```python
from build123d import *

# Parameters (mm, degrees)
SKETCH1_W                        = 125
SKETCH1_H                        = 120
TEST_BASE_POSTION_DEPTH          = 11.215
SKETCH8_R                        = 20.5
FINGER_GEARS_DEPTH               = 7
SKETCH9_R                        = 10.5
INTERMEDIATE_GEAR_DEPTH          = 7
SKETCH11_R                       = 18.5
XL320_FINGER_KNUCKLE_MOUNT_DEPTH = 7
SKETCH10_R                       = 15.5
CONNECT_FINGER_HOLES_DEPTH       = 88.361468766
THUMB_MOUNT_HOLES_R              = 2.25
THUMB_MOUNT_HOLES_M4_DEPTH       = 88.361468766
SKETCH16_R                       = 2.25
FINGERS_MOUNT_HOLES_M4_DEPTH     = 88.361468766
SKETCH17_R                       = 3.25
CONNECT_HOLES_M6_DEPTH           = 88.361468766
SKETCH18_R                       = 3.75
NUTS_M4_DEPTH                    = 4
SKETCH19_R                       = 5.25
NUTS_M6_DEPTH                    = 6


with BuildPart() as part:
    # Sketch1 → Test_Base_Postion (new body)
    with BuildSketch(Plane(origin=(0, 0, 0), x_dir=(1, 0, 0), z_dir=(0, 1, 0))):
        Rectangle(SKETCH1_W, SKETCH1_H)
    extrude(amount=TEST_BASE_POSTION_DEPTH)

    # Sketch8 → Finger_Gears (cut)
    with BuildSketch(Plane(origin=(0, 11.215, 0), x_dir=(1, 0, 0), z_dir=(0, 1, 0))):
        with Locations((-25.25, -19)):
            Circle(SKETCH8_R)
        with Locations((-25.25, 19)):
            Circle(SKETCH8_R)
    extrude(amount=-FINGER_GEARS_DEPTH, mode=Mode.SUBTRACT)

    # Sketch9 → Intermediate_Gear (cut)
    with BuildSketch(Plane(origin=(0, 11.215, 0), x_dir=(1, 0, 0), z_dir=(0, 1, 0))):
        with Locations((0.646123438, -8.351488795)):
            Circle(SKETCH9_R)
    extrude(amount=-INTERMEDIATE_GEAR_DEPTH, mode=Mode.SUBTRACT)

    # Sketch11 → XL320_Finger_Knuckle_Mount (cut)
    with BuildSketch(Plane(origin=(0, 11.215, 0), x_dir=(1, 0, 0), z_dir=(0, 1, 0))):
        with Locations(Location((42, 0, 0), (0, 0, 270))):
            Circle(SKETCH11_R)
    extrude(amount=-XL320_FINGER_KNUCKLE_MOUNT_DEPTH, mode=Mode.SUBTRACT)

    # Sketch10 → Connect_Finger_Holes (cut, through all)
    with BuildSketch(Plane(origin=(0, 11.215, 0), x_dir=(1, 0, 0), z_dir=(0, 1, 0))):
        with Locations(Location((-25.25, 19, 0), (0, 0, 270))):
            Circle(SKETCH10_R)
        with Locations(Location((-25.25, -19, 0), (0, 0, 270))):
            Circle(SKETCH10_R)
        with Locations(Location((42, 0, 0), (0, 0, 270))):
            Circle(SKETCH10_R)
    extrude(amount=-CONNECT_FINGER_HOLES_DEPTH, mode=Mode.SUBTRACT)

    # Thumb_Mount_Holes → Thumb_Mount_Holes_(M4) (cut, through all)
    with BuildSketch(Plane(origin=(0, 11.215, 0), x_dir=(1, 0, 0), z_dir=(0, 1, 0))):
        with Locations(Location((21.5, 44.5, 0), (0, 0, 270))):
            Circle(THUMB_MOUNT_HOLES_R)
        with Locations(Location((42, 53.5, 0), (0, 0, 270))):
            Circle(THUMB_MOUNT_HOLES_R)
        with Locations(Location((48, -24, 0), (0, 0, 270))):
            Circle(THUMB_MOUNT_HOLES_R)
        with Locations(Location((36, -24, 0), (0, 0, 270))):
            Circle(THUMB_MOUNT_HOLES_R)
    extrude(amount=-THUMB_MOUNT_HOLES_M4_DEPTH, mode=Mode.SUBTRACT)

    # Sketch16 → Fingers_Mount_Holes_(M4) (cut, through all)
    with BuildSketch(Plane(origin=(0, 11.215, 0), x_dir=(1, 0, 0), z_dir=(0, 1, 0))):
        with Locations(Location((11.5, 41, 0), (0, 0, 270))):
            Circle(SKETCH16_R)
        with Locations(Location((11.5, -41, 0), (0, 0, 270))):
            Circle(SKETCH16_R)
        with Locations(Location((-53, 6, 0), (0, 0, 270))):
            Circle(SKETCH16_R)
        with Locations(Location((-53, -6, 0), (0, 0, 270))):
            Circle(SKETCH16_R)
    extrude(amount=-FINGERS_MOUNT_HOLES_M4_DEPTH, mode=Mode.SUBTRACT)

    # Sketch17 → Connect_Holes_(M6) (cut, through all)
    with BuildSketch(Plane(origin=(0, 11.215, 0), x_dir=(1, 0, 0), z_dir=(0, 1, 0))):
        with Locations(Location((-52.5, 50, 0), (0, 0, 270))):
            Circle(SKETCH17_R)
        with Locations(Location((-52.5, -50, 0), (0, 0, 270))):
            Circle(SKETCH17_R)
        with Locations(Location((52.5, -50, 0), (0, 0, 270))):
            Circle(SKETCH17_R)
    extrude(amount=-CONNECT_HOLES_M6_DEPTH, mode=Mode.SUBTRACT)

    # Sketch18 → Nuts_(M4) (cut)
    with BuildSketch(Plane.XZ):
        with Locations(Location((11.5, 41, 0), (0, 0, 270))):
            Circle(SKETCH18_R)
        with Locations(Location((11.5, -41, 0), (0, 0, 270))):
            Circle(SKETCH18_R)
        with Locations(Location((21.5, -44.5, 0), (0, 0, 270))):
            Circle(SKETCH18_R)
        with Locations(Location((42, -53.5, 0), (0, 0, 270))):
            Circle(SKETCH18_R)
    extrude(amount=-NUTS_M4_DEPTH, mode=Mode.SUBTRACT)

    # Sketch19 → Nuts_(M6) (cut)
    with BuildSketch(Plane.XZ):
        with Locations(Location((-52.5, 50, 0), (0, 0, 270))):
            Circle(SKETCH19_R)
        with Locations(Location((52.5, 50, 0), (0, 0, 270))):
            Circle(SKETCH19_R)
        with Locations(Location((-52.5, -50, 0), (0, 0, 270))):
            Circle(SKETCH19_R)
    extrude(amount=-NUTS_M6_DEPTH, mode=Mode.SUBTRACT)


solid = part.part
```
Check sheet for the modelled part. Datum: model origin and axes. Units: mm. A direction names the side the tool comes from. Round coordinates to 2 decimals unless told otherwise and drop trailing zeros. Loops run counter-clockwise (first coordinate to the right, second up) from the corner with the lowest first, then second, coordinate; pieces in that order, holes last. Notation, with made-up numbers: M 52,21.5 L 86,21.5 A21 cw 86,27.5 Z; hole C 2.25,52.5 d3. An arc over 180 degrees is marked long. Answer as a JSON object with one key per item and string values.
1. Section check D-D (y = 7.5). State how many separate pieces and enclosed holes the cut face has, plus the area to 3 significant figures.
Reply:
{"separate pieces": "1", "enclosed holes": "13", "area": "10,800 mm²"}
2. Section check C-C (x = -25.25). Record the boundary of the cut face in (y, z) (3 decimals).
Reply:
{"outline": "M 0,-60 L 11.215,-60 L 11.215,-39.5 L 4.215,-39.5 L 4.215,-34.5 L 0,-34.5 Z; M 0,-3.5 L 4.215,-3.5 L 4.215,3.5 L 0,3.5 Z; M 0,34.5 L 4.215,34.5 L 4.215,39.5 L 11.215,39.5 L 11.215,60 L 0,60 Z"}
3. Scan lines: line 1 (X direction, y = 7.85, z = 50); line 2 (Z direction, x = -26, y = 2.75); line 3 (X direction, y = 3.2, z = -19). Record each from-to range of solid material in increasing order.
Reply:
{"line 1": "x = -62.5 to -55.75, -49.25 to 49.25, 55.75 to 62.5", "line 2": "z = -60 to -34.48, -3.52 to 3.52, 34.48 to 60", "line 3": "x = -62.5 to -40.75, -9.75 to 62.5"}
4. Section check B-B (z = 41). Record the boundary of the cut face in (x, y) (3 decimals).
Reply:
{"outline": "M -62.5,0 L 7.75,0 L 7.75,4 L 9.25,4 L 9.25,11.215 L -62.5,11.215 Z; M 13.75,4 L 15.25,4 L 15.25,0 L 62.5,0 L 62.5,11.215 L 13.75,11.215 Z"}
5. Mould release check, pull along X, two halves, no side actions. Record for faces 1 (the flat face through (-1, 6, -60)), 2 (the flat face through (-62.5, 6, 1)), 3 (the flat face through (-20, 4.215, 0)), 4 (the cylindrical face through (-53.745, 8.644, 53.002)): pulls with the +X half, pulls with the -X half, needs draft (parallel to the pull), parting line crosses it, or undercut.
Reply:
{"face 1": "needs draft", "face 2": "pulls with the -X half", "face 3": "undercut", "face 4": "undercut"}
6. Gauge pin test, flat end, axial feed: P1, Ø8.5, axis at x = 52.5, z = 50, coming from the -Y side. Record the tip position at first contact, or that the pin passes through.
Reply:
{"P1": "stops at y = 6"}
7. Section check A-A (x = 21.5). Record the boundary of the cut face in (y, z) (3 decimals), plus the area to 3 significant figures.
Reply:
{"outline": "M 0,-60 L 11.215,-60 L 11.215,-46.75 L 4,-46.75 L 4,-48.25 L 0,-48.25 Z; M 0,-40.75 L 4,-40.75 L 4,-42.25 L 11.215,-42.25 L 11.215,60 L 0,60 Z", "area": "1,280 mm²"}
8. Access from +Z, -Z, +X, -X, +Y, -Y to the whole of each face (thin tool, end or side, straight path). Record for faces 5 (the cylindrical face through (-36.531, 7.764, 36.117)), 6 (the cylindrical face through (51.255, 8.644, 53.002)), 7 (the flat face through (10, 4, -43)).
Reply:
{"face 5": "+Y", "face 6": "+Y, -Y", "face 7": "-Y"}
